from build123d import *

# Parameters (mm, degrees)
SKETCH_5_R               = 1.925
CUT_EXTRUDE_3_DEPTH      = 6.5
PATTERN_CIRCULAR_1_COUNT = 3
CUT_EXTRUDE_4_REACH      = 100.655
SKETCH_6_R               = 10.15
CHAMFER_1_SIZE           = 1
CHAMFER_2_SIZE           = 0.5
CHAMFER_3_SIZE           = 3
CHAMFER_3_SIZE2          = 3.645101124


with BuildPart() as part:
    # 스케치2 → 회전1 (revolve)
    with BuildSketch(Plane(origin=(0, 0, 0), x_dir=(0, 0, -1), z_dir=(1, 0, 0)), mode=Mode.PRIVATE) as revolve_1_sk:
        Polygon((0.919706719, -10.18531024), (0, -10.2), (0, -17.5), (70, -17.5), (110, -14), (190, -14), (190, 0), (95.5, 0), (95.5, -7.175), (79.5, -7.175), (72, -9.05), align=None)
    revolve(revolve_1_sk.sketch.rotate(Axis((0, 0, 0), (0, 0, -1)), 270), axis=Axis((0, 0, 0), (0, 0, -1)))

    # 스케치5 → 컷-돌출3 (cut)
    with BuildSketch(Plane(origin=(0, -17.5, 0), x_dir=(-1, 0, 0), z_dir=(0, -1, 0))):
        with Locations(Location((0, 30, 0), (0, 0, 90))):
            Circle(SKETCH_5_R)
        with Locations(Location((0, 65, 0), (0, 0, 90))):
            Circle(SKETCH_5_R)
    cut_extrude_3 = extrude(amount=-CUT_EXTRUDE_3_DEPTH, mode=Mode.SUBTRACT)

    # 원형 패턴1: 컷-돌출3 ×3 about axis
    pattern_circular_1_axis = Axis((0, 0, 0), (0, 0, 1))
    for i in range(1, PATTERN_CIRCULAR_1_COUNT):
        add(cut_extrude_3.rotate(pattern_circular_1_axis, i * 360 / PATTERN_CIRCULAR_1_COUNT), mode=Mode.SUBTRACT)

    # 스케치6 → 컷-돌출4 (cut, up to next)
    with BuildSketch(Plane.XY.offset(-95.5), mode=Mode.PRIVATE) as cut_extrude_4_sk1:
        Circle(SKETCH_6_R)
    cut_extrude_4_tool1 = extrude(cut_extrude_4_sk1.sketch, amount=-CUT_EXTRUDE_4_REACH, mode=Mode.PRIVATE) & part.part
    add(cut_extrude_4_tool1.solids().sort_by_distance((0, 0, -95.5))[0], mode=Mode.SUBTRACT)

    # 모따기1
    chamfer_1_edges = [part.edges().sort_by_distance(p)[0] for p in [
        (-14, 0, -190),
    ]]
    chamfer(chamfer_1_edges, length=CHAMFER_1_SIZE)

    # 모따기2
    chamfer_2_edges = [part.edges().sort_by_distance(p)[0] for p in [
        (-10.15, 0, -190),
    ]]
    chamfer(chamfer_2_edges, length=CHAMFER_2_SIZE)

    # 모따기3
    chamfer_3_edges = [part.edges().sort_by_distance(p)[0] for p in [
        (-10.2, 0, 0),
    ]]
    chamfer_3_side = [part.faces().sort_by_distance(p)[0] for p in [
        (-10.694974747, 0, 0),
    ]]
    chamfer(chamfer_3_edges, length=CHAMFER_3_SIZE, length2=CHAMFER_3_SIZE2, reference=chamfer_3_side[0])


solid = part.part
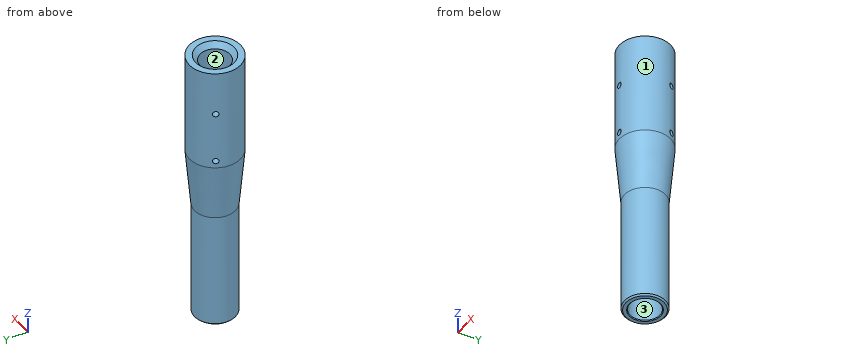
Part model, mm, in its own coordinate system. Face numbers are marked on the shaded views. Coordinates: 2 decimals unless noted, no trailing zeros. Write each loop counter-clockwise with the first axis right and the second up, starting at its lowest first coordinate (ties: lowest second). Pieces come first, ordered by that corner, then holes. Notation, with made-up numbers: M 46,19 L 103,19 A23 ccw 103,40 Z; hole C -32,31 d4. An arc over 180 degrees is marked long. Return JSON: item names as keys, results as strings.
1. Pull direction X, two halves, no side cores. Call the marked faces 1, 2 and 3: pulls with the +X half, pulls with the -X half, needs draft (parallel to the pull), parting line crosses it, or undercut.
Determined:
{"face 1": "parting line crosses it", "face 2": "undercut", "face 3": "undercut"}
2. Flat gauge pins, fed straight in: pin 1 Ø3 at (x, z) = (0, -65.5) entering from -Y; pin 2 Ø3.5 at (x, z) = (0, -30) entering from -Y; pin 3 Ø16 at (x, y) = (0, 0) entering from -Z; pin 4 Ø8.5 at (x, y) = (0, 0) entering from -Z. Where does each tip first touch, or does it go through?
Determined:
{"pin 1": "y = -17.5", "pin 2": "y = -11", "pin 3": "z = -95.5", "pin 4": "through"}
3. Probe L1, parallel to Y at x = 0, z = -157.5; L2, parallel to Z at x = 0, y = -13 (3 decimals); L3, parallel to Z at x = 0, y = -13.5 (3 decimals). List the from-to ranges inside material, lowest first.
Determined:
{"L1": "-14 to -10.15, 10.15 to 14", "L2": "-190 to -66.925, -63.075 to -31.925, -28.075 to -0.238", "L3": "-189.5 to -66.925, -63.075 to -31.925, -28.075 to 0"}
4. Saw through at A-A, the plane z = -30. Write the cut outline in (x, y) (3 decimals).
Determined:
{"outline": "M -16.026,7.03 A17.5 ccw -1.925,-17.394 L -1.925,-11 L 1.925,-11 L 1.925,-17.394 A17.5 ccw 16.026,7.03 L 10.489,3.833 L 8.564,7.167 L 14.101,10.364 A17.5 ccw -14.101,10.364 L -8.564,7.167 L -10.489,3.833 Z; hole C 0,0 d19.442"}
5. Saw through at B-B, the plane z = -65. Write the cut outline in (x, y) (3 decimals).
Determined:
{"outline": "M -16.026,7.03 A17.5 ccw -1.925,-17.394 L -1.925,-11 L 1.925,-11 L 1.925,-17.394 A17.5 ccw 16.026,7.03 L 10.489,3.833 L 8.564,7.167 L 14.101,10.364 A17.5 ccw -14.101,10.364 L -8.564,7.167 L -10.489,3.833 Z; hole C 0,0 d18.324"}
6. Saw through at C-C, the plane z = -175.5. Write the cut outline in (x, y).
Determined:
{"outline": "C 0,0 d28; hole C 0,0 d20.3"}
